Source: three-view drawing plus pictorial views. Frame: mm from the lowest corner of the part. A direction names the side the tool comes from. Coordinates: 2 decimals unless noted, no trailing zeros. Write each loop counter-clockwise with the first axis right and the second up, starting at its lowest first coordinate (ties: lowest second). Pieces come first, ordered by that corner, then holes. Notation, with made-up numbers: M 37,1 L 52,1 A18 ccw 52,14 Z; hole C 79,-33 d6. An arc over 180 degrees is marked long. Write item = value, one per line. Start each with the question number.
Item 1: Section C-C on y = 6.75. Output: boundary loops of the cut face in (x, z), plus the area to 3 significant figures.
Item 2: Ray query, L1, parallel to Y at x = 12.7, z = 9.75; L2, parallel to X at y = 4.75, z = 5.25; L3, parallel to X at y = 21.75, z = 18.75. Return the intervals inside material, ascending. Write a range as [from, to].
Item 3: Section A-A on y = 22.75. Output: boundary loops of the cut face in (x, z), plus the area to 3 significant figures.
Item 4: First-contact query: pin 1 Ø4 at (x, z) = (19.5, 15.5) entering from -Y; pin 2 Ø3.5 at (x, z) = (12, 9) entering from -Y; pin 3 Ø1.5 at (y, z) = (10.5, 12.5) entering from -X; pin 4 Ø1.5 at (x, y) = (5.5, 14.5) entering from +Z. Flat tips, straight axial feed; report the tip coordinate or a pass-through.
Item 5: Section B-B on x = 12.7. Output: boundary loops of the cut face in (y, z).
Item 6: Reachability of the marked faces 5, 6, 7, 8 and 9 from +Z, -Z, +X, -X, +Y, -Y: full face, straight path, thin tool, end or side. Return the list, or none.
Item 7: Pull-direction query (Y, two-part tool) for the marked faces 1, 2, 3 and 4; classes: +Y half, -Y half, draft (parallel to the pull), parting line (faces both ways), or undercut.
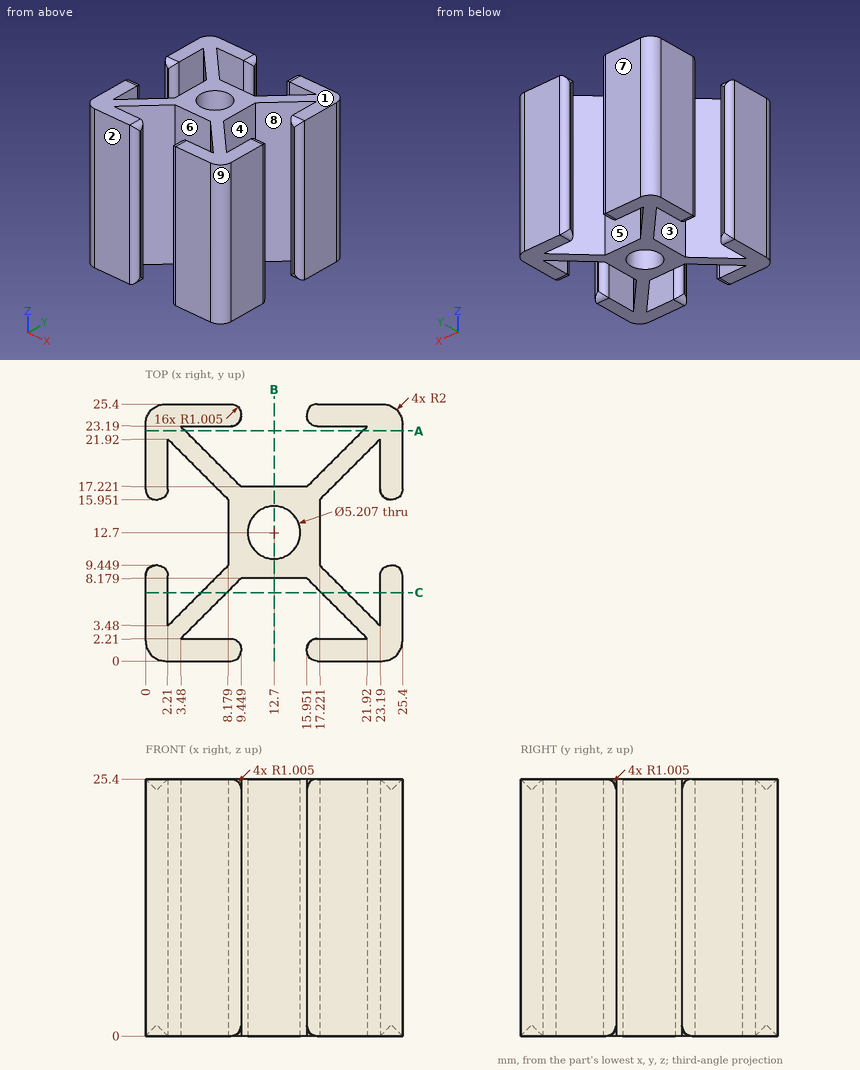
Responses:
q1.outline = M 0,0 L 2.21,0 L 2.21,25.4 L 0,25.4 Z; M 5.48,0 L 8.02,0 L 8.02,25.4 L 5.48,25.4 Z; M 17.38,0 L 19.92,0 L 19.92,25.4 L 17.38,25.4 Z; M 23.19,0 L 25.4,0 L 25.4,25.4 L 23.19,25.4 Z
q1.area = 241 mm²
q2.L1 = [8.18, 10.1], [15.3, 17.22]
q2.L2 = [0, 2.21], [3.48, 6.02], [19.38, 21.92], [23.19, 25.4]
q2.L3 = [0, 2.21], [2.38, 4.92], [20.48, 23.02], [23.19, 25.4]
q3.outline = M 0,0 L 3.92,0 L 3.92,25.4 L 0,25.4 Z; M 21.48,0 L 25.4,0 L 25.4,25.4 L 21.48,25.4 Z
q3.area = 199 mm²
q4.pin_1 = 0
q4.pin_2 = 8.18
q4.pin_3 = 8.18
q4.pin_4 = through
q5.outline = M 8.18,0 L 10.1,0 L 10.1,25.4 L 8.18,25.4 Z; M 15.3,0 L 17.22,0 L 17.22,25.4 L 15.3,25.4 Z
q6.face_5 = +Z, -Z, +Y
q6.face_6 = +Z, -Z, -Y
q6.face_7 = +Z, -Z, +X, -X, +Y
q6.face_8 = +Z, -Z
q6.face_9 = +Z, -Z, +X, -Y
q7.face_1 = draft
q7.face_2 = -Y half
q7.face_3 = undercut
q7.face_4 = undercut
